For this review, use the dimensioned drawing (mm, ordinates from the lowest corner) and the shaded views. Give positions to 0.01 mm unless a question says otherwise; leave off trailing zeros. Write each question's results on one line, items separated by ' | '. Start each with the question number.
Q1. Mouldability with a two-part tool opening along Z and no side actions: class the marked faces 1, 2 and 3 as released by +Z, released by -Z, zero draft, split by the parting line, or undercut.
Q2. Wall thickness on L1, parallel to Y at x = 42, z = 38.5 (1 decimal); L2, parallel to X at y = 7.75, z = 33.5 (1 decimal); L3, parallel to Y at x = 69, z = 18 (1 decimal): over which ranges is each line inside the solid? List them lowest first. Write a range as [from, to].
Q3. Insertion check: pin 1 Ø8 at (x, z) = (36, 37.5) entering from -Y (1 decimal); pin 2 Ø1 at (y, z) = (10, 32.5) entering from +X (1 decimal). Each pin has a flat end and moves straight along its axis. Give the tip position at first contact, or say it passes through.
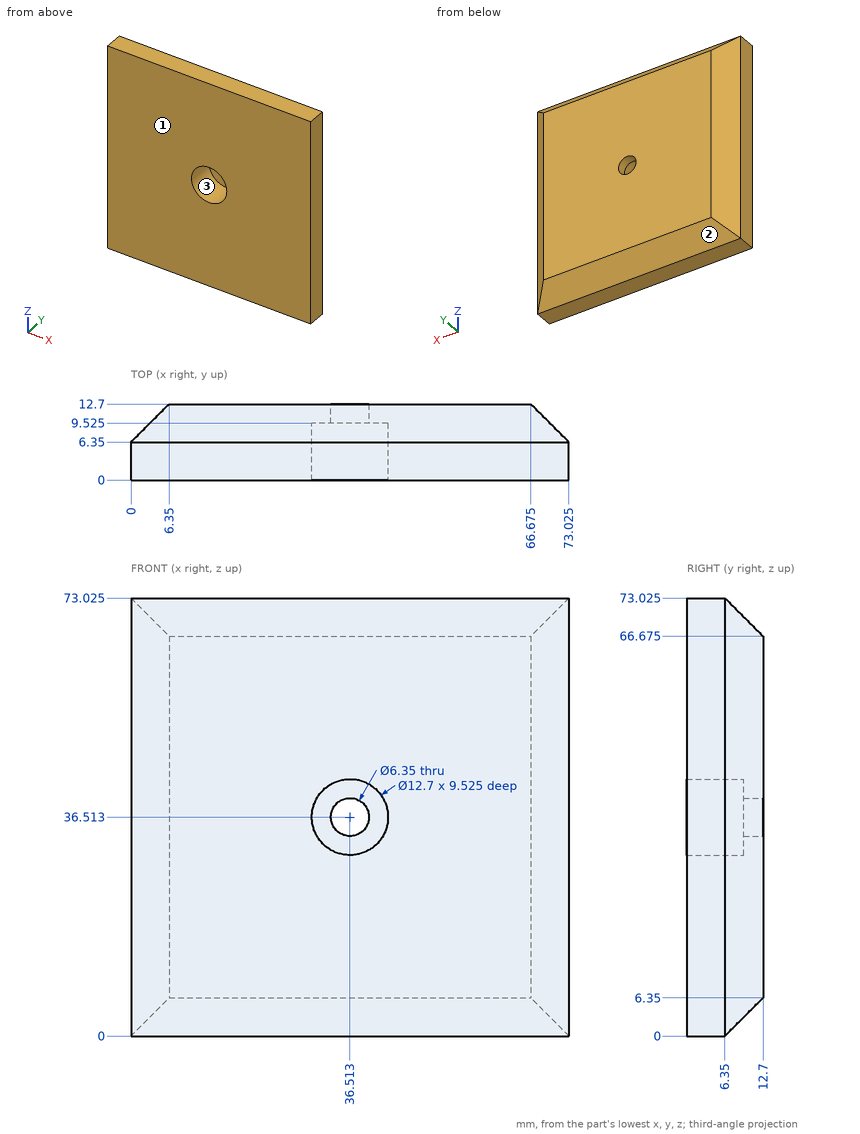
Output:
1) face 1: zero draft | face 2: released by -Z | face 3: undercut
2) L1: [9.5, 12.7] | L2: [1.4, 30.9], [42.1, 71.6] | L3: [0, 10.4]
3) pin 1: y = 9.5 | pin 2: x = 69.9
